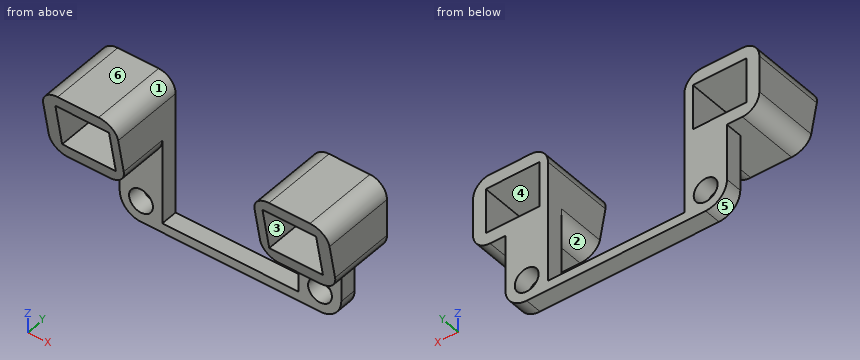
```python
from build123d import *

# Parameters (mm, degrees)
SKETCH1_R           = 1.4
BOSS_EXTRUDE1_DEPTH = 2
FILLET1_R           = 2.5
SKETCH2_W           = 8.8
SKETCH2_H           = 8.3
SKETCH2_W_2         = 6.3
SKETCH2_H_2         = 5.3
BOSS_EXTRUDE2_DEPTH = 9
CUT_EXTRUDE1_DEPTH  = 36.921024484
FILLET2_R           = 2


with BuildPart() as part:
    # Sketch1 → Boss-Extrude1 (new body)
    with BuildSketch(Plane(origin=(0, 0, 0), x_dir=(1, 0, 0), z_dir=(0, 1, 0))):
        Polygon((-13, 0), (-13, 10.6), (13, 10.6), (13, 0), (8, 0), (8, 9.5), (-8, 9.5), (-8, 0), align=None)
        with Locations(Location((-10.5, 8.1, 0), (0, 0, 270))):
            Circle(SKETCH1_R, mode=Mode.SUBTRACT)
        with Locations(Location((10.5, 8.1, 0), (0, 0, 270))):
            Circle(SKETCH1_R, mode=Mode.SUBTRACT)
    extrude(amount=BOSS_EXTRUDE1_DEPTH)

    # Fillet1
    fillet1_edges = [part.edges().sort_by_distance(p)[0] for p in [
        (-13, 1, -10.6),
        (13, 1, -10.6),
    ]]
    fillet(fillet1_edges, radius=FILLET1_R)

    # Sketch2 → Boss-Extrude2 (add)
    # profile 1 of 2: a face of its own
    with BuildSketch(Plane(origin=(0, 2, 0), x_dir=(1, 0, 0), z_dir=(0, 1, 0))):
        with Locations((-12.4, -2.65)):
            Rectangle(SKETCH2_W, SKETCH2_H)
        with Locations((-12.15, -2.65)):
            Rectangle(SKETCH2_W_2, SKETCH2_H_2, mode=Mode.SUBTRACT)
    # profile 2 of 2: a face of its own
    with BuildSketch(Plane(origin=(0, 2, 0), x_dir=(1, 0, 0), z_dir=(0, 1, 0))):
        with Locations((12.4, -2.65)):
            Rectangle(SKETCH2_W, SKETCH2_H)
        with Locations((12.15, -2.65)):
            Rectangle(SKETCH2_W_2, SKETCH2_H_2, mode=Mode.SUBTRACT)
    extrude(amount=-BOSS_EXTRUDE2_DEPTH)

    # Sketch3 → Cut-Extrude1 (cut, through all)
    with BuildSketch(Plane.ZY.offset(16.8)):
        Polygon((-37.097656143, -7), (-1.5, -7), (6.8, -7), (-1.5, -5.39), (-36.44627134, 1.388734561), (-107.427912809, 6.900455328), (-108.079297611, -1.488279233), align=None)
    extrude(amount=-CUT_EXTRUDE1_DEPTH, mode=Mode.SUBTRACT)

    # Fillet2
    fillet2_edges = [part.edges().sort_by_distance(p)[0] for p in [
        (16.8, -1.695, -1.5),
        (8, -2.695, -1.5),
        (-8, -2.695, -1.5),
        (-16.8, -1.695, -1.5),
        (-16.8, -2.5, 6.8),
        (-8, -2.5, 6.8),
        (16.8, -2.5, 6.8),
        (8, -2.5, 6.8),
    ]]
    fillet(fillet2_edges, radius=FILLET2_R)


solid = part.part
```
Here's how the part is built. I have some questions about the finished solid (model axes, mm). Face numbers are marked on the shaded views. A direction names the side the tool comes from. Round coordinates to 2 decimals unless told otherwise and drop trailing zeros. Order: outer loops, then holes, each group sorted by start corner. A loop starts at its lowest first (then second) coordinate and runs counter-clockwise, first axis right, second up. Notation, with made-up numbers: (-30, 22.5) -> (7, 22.5) arc R7 cw to (7, 30.5) -> close; hole circle Ø11 at (35, 3). An arc over 180 degrees is marked (long way). Use a Markdown table: item, result. Add a question column.
(1) For pin 1 Ø2 at (x, z) = (-10.5, -8.1) entering from +Y; pin 2 Ø1.6 at (y, z) = (1, -5.5) entering from -X; pin 3 Ø9 at (x, z) = (-4, -3.5) entering from -Y; pin 4 Ø5 at (x, y) = (-13, -2) entering from -Z, each with a flat end and sliding along its axis, tell me the tip position at first contact or that it passes through.
(2) I need wall thicknesses on line 1 along X through (y, z) = (0.5, -8.1); line 2 along X through (y, z) = (-4.5, 1); line 3 along X through (y, z) = (1, -4). Which ranges of each line are inside material? Lowest first, please.
(3) If we mould it in two halves opening along Z, with no side actions, what happens to the marked faces 4, 5 and 6? For each: released by +Z, released by -Z, zero draft, split by the parting line, or undercut.
(4) Suppose I cut it at B-B, the plane x = -14. Please give me the cut outline in (y, z), and give its area (3 significant figures).
(5) For the marked faces 1, 2 and 3, which set-ups out of +Z, -Z, +X, -X, +Y, -Y let a thin tool reach every point of the face, with its end or its side?
(6) Suppose I cut it at D-D, the plane x = 11.5. Please give me the cut outline in (y, z).
(7) Suppose I cut it at A-A, the plane y = -2.25. Please give me the cut outline in (x, z), and give its area (3 significant figures).
(8) Suppose I cut it at C-C, the plane z = 2.25. Please give me the cut outline in (x, y), and give its area (3 significant figures).
Verdict:
| question | item | result |
|---|---|---|
| 1 | pin 1 | through |
| 1 | pin 2 | x = -13 |
| 1 | pin 3 | y = 0 |
| 1 | pin 4 | z = -10.39 |
| 2 | line 1 | -13 to -11.9, -9.1 to -8, 8 to 9.1, 11.9 to 13 |
| 2 | line 2 | -16.8 to -15.3, -9 to -8, 8 to 9, 15.3 to 16.8 |
| 2 | line 3 | -13 to -8, 8 to 13 |
| 3 | face 4 | undercut |
| 3 | face 5 | released by -Z |
| 3 | face 6 | released by +Z |
| 4 | outline | (-7, 6.8) -> (-6.71, 5.3) -> (2, 5.3) -> (2, 6.8) -> close; (-5.68, 0) -> (-5.39, -1.5) -> (2, -1.5) -> (2, 0) -> close |
| 4 | area | 24.6 mm2 |
| 5 | face 1 | +Z, +Y, -Y |
| 5 | face 2 | -Z, -Y |
| 5 | face 3 | +Y, -Y |
| 6 | outline | (-7, 6.8) -> (-6.71, 5.3) -> (2, 5.3) -> (2, 6.8) -> close; (-5.68, 0) -> (-5.39, -1.5) -> (0, -1.5) -> (0, -7.12) -> (2, -7.12) -> (2, 0) -> close; (0, -10.39) -> (2, -10.39) -> (2, -9.08) -> (0, -9.08) -> close |
| 7 | outline | (-16.8, 0.5) arc R2 ccw to (-14.8, -1.5) -> (-10, -1.5) arc R2 ccw to (-8, 0.5) -> (-8, 4.8) arc R2 ccw to (-10, 6.8) -> (-14.8, 6.8) arc R2 ccw to (-16.8, 4.8) -> close; (8, 0.5) arc R2 ccw to (10, -1.5) -> (14.8, -1.5) arc R2 ccw to (16.8, 0.5) -> (16.8, 4.8) arc R2 ccw to (14.8, 6.8) -> (10, 6.8) arc R2 ccw to (8, 4.8) -> close; hole (-15.3, 0) -> (-9, 0) -> (-9, 5.3) -> (-15.3, 5.3) -> close; hole (9, 0) -> (15.3, 0) -> (15.3, 5.3) -> (9, 5.3) -> close |
| 7 | area | 72.4 mm2 |
| 8 | outline | (-16.8, -6.12) -> (-15.3, -6.12) -> (-15.3, 2) -> (-16.8, 2) -> close; (-9, -6.12) -> (-8, -6.12) -> (-8, 2) -> (-9, 2) -> close; (8, -6.12) -> (9, -6.12) -> (9, 2) -> (8, 2) -> close; (15.3, -6.12) -> (16.8, -6.12) -> (16.8, 2) -> (15.3, 2) -> close |
| 8 | area | 40.6 mm2 |
